```python
from build123d import *

# Parameters (mm, degrees)
EXTRUDE_THIN1_DEPTH = 10
FILLET1_R           = 0.5


with BuildPart() as part:
    # Sketch1 → Extrude-Thin1 (new body)
    with BuildSketch(Plane(origin=(0, 0, 0), x_dir=(1, 0, 0), z_dir=(0, 1, 0))):
        with BuildLine():
            ThreePointArc((31.228009552, -30.556896247), (17.805759331, -35.661082732), (3.450021006, -36.010793734))
            ThreePointArc((3.450021006, -36.010793734), (0.781528732, -34.960126351), (-1.143442514, -32.834276246))
            Line((-1.143442514, -32.834276246), (-11.514158233, -14.115081405))
            ThreePointArc((-11.514158233, -14.115081405), (-11.864920764, -12.594591782), (-11.35681344, -11.119210477))
            Line((-11.35681344, -11.119210477), (0, 5.1))
            Line((0, 5.1), (0, 0))
            Line((0, 0), (30, 0))
            Line((30, 0), (30, 5.1))
            Line((30, 5.1), (36.395958363, 2.511232605))
            ThreePointArc((36.395958363, 2.511232605), (37.463728778, 1.925417586), (38.366240646, 1.107624688))
            Line((38.366240646, 1.107624688), (42.902523658, -4.091619145))
            ThreePointArc((42.902523658, -4.091619145), (43.590417547, -5.096663868), (44.026071732, -6.233993339))
            Line((44.026071732, -6.233993339), (45.723869414, -12.921854211))
            ThreePointArc((45.723869414, -12.921854211), (45.883457457, -14.129266548), (45.7582513, -15.340726954))
            Line((45.7582513, -15.340726954), (44.251223786, -22.074141249))
            ThreePointArc((44.251223786, -22.074141249), (43.848071102, -23.223393532), (43.189020782, -24.247583736))
            Line((43.189020782, -24.247583736), (38.802344779, -29.573658617))
            ThreePointArc((38.802344779, -29.573658617), (37.883123065, -30.501625481), (36.810104599, -31.246422387))
            Line((36.810104599, -31.246422387), (28.716751538, -35.827648886))
            ThreePointArc((28.716751538, -35.827648886), (23.339920043, -38.206219709), (17.601311476, -39.485394366))
            ThreePointArc((17.601311476, -39.485394366), (9.20703571, -39.890619172), (0.842295428, -39.078712278))
            Line((0.842295428, -39.078712278), (1.179197641, -37.107292257))
            ThreePointArc((1.179197641, -37.107292257), (9.255554358, -37.891207773), (17.360428291, -37.499953535))
            ThreePointArc((17.360428291, -37.499953535), (22.714760553, -36.306436666), (27.731541539, -34.087142851))
            Line((27.731541539, -34.087142851), (35.824894599, -29.505916352))
            ThreePointArc((35.824894599, -29.505916352), (36.597062561, -28.969943927), (37.258554958, -28.302158326))
            Line((37.258554958, -28.302158326), (41.645230962, -22.976083445))
            ThreePointArc((41.645230962, -22.976083445), (42.051182062, -22.345219415), (42.299509498, -21.63732168))
            Line((42.299509498, -21.63732168), (43.806537012, -14.903907385))
            ThreePointArc((43.806537012, -14.903907385), (43.883659464, -14.157691701), (43.785359016, -13.413969481))
            Line((43.785359016, -13.413969481), (42.087561335, -6.72610861))
            ThreePointArc((42.087561335, -6.72610861), (41.819214153, -6.025554893), (41.39549646, -5.406483786))
            Line((41.39549646, -5.406483786), (36.859213448, -0.207239953))
            ThreePointArc((36.859213448, -0.207239953), (36.303298861, 0.29649082), (35.645591002, 0.657331631))
            Line((35.645591002, 0.657331631), (32, 2.13288644))
            Line((32, 2.13288644), (32, -2))
            Line((32, -2), (-2, -2))
            Line((-2, -2), (-2, -1.243189605))
            Line((-2, -1.243189605), (-9.718509351, -12.26636335))
            ThreePointArc((-9.718509351, -12.26636335), (-9.867673478, -12.69948831), (-9.764700771, -13.145855637))
            Line((-9.764700771, -13.145855637), (0.606014947, -31.865050477))
            ThreePointArc((0.606014947, -31.865050477), (1.919083649, -33.31514343), (3.73932574, -34.031828659))
            ThreePointArc((3.73932574, -34.031828659), (17.420438321, -33.698551784), (30.211930629, -28.834228658))
            Line((30.211930629, -28.834228658), (31.228009552, -30.556896247))
        make_face()
    extrude(amount=EXTRUDE_THIN1_DEPTH)

    # Fillet1
    fillet1_edges = [part.edges().sort_by_distance(p)[0] for p in [
        (0, 5, -5.1),
        (30, 5, -5.1),
    ]]
    fillet(fillet1_edges, radius=FILLET1_R)


solid = part.part
```
Read the model definition and answer for the solid it produces. Units are mm, in the model's axes. A direction names the side the tool comes from. Coordinates: 2 decimals unless noted, no trailing zeros. Loops run counter-clockwise (first coordinate to the right, second up) from the corner with the lowest first, then second, coordinate; pieces in that order, holes last. Notation, with made-up numbers: (41, 5.5) -> (93, 5.5) arc R14 ccw to (93, 15.5) -> close; hole circle Ø4 at (84, 20). An arc over 180 degrees is marked (long way). Return JSON: item names as keys, results as strings.
Item 1: Find section A-A (x = 6.5). Determine the outline of the cut face in (y, z), plus the area to 3 significant figures.
Answers:
{"outline": "(0, 0) -> (10, 0) -> (10, 2) -> (0, 2) -> close; (0, 34.34) -> (10, 34.34) -> (10, 36.34) -> (0, 36.34) -> close; (0, 37.76) -> (10, 37.76) -> (10, 39.76) -> (0, 39.76) -> close", "area": "60.1 mm2"}
Item 2: Find section B-B (z = 17). Determine the outline of the cut face in (x, y), plus the area to 3 significant figures.
Answers:
{"outline": "(-9.92, 0) -> (-7.63, 0) -> (-7.63, 10) -> (-9.92, 10) -> close; (43.34, 0) -> (45.39, 0) -> (45.39, 10) -> (43.34, 10) -> close", "area": "43.4 mm2"}
Item 3: Find section C-C (x = -4). Determine the outline of the cut face in (y, z).
Answers:
{"outline": "(0, 0.61) -> (10, 0.61) -> (10, 4.1) -> (0, 4.1) -> close; (0, 23.55) -> (10, 23.55) -> (10, 27.68) -> (0, 27.68) -> close"}
Item 4: For a pull along X with two mould halves and no side action, classify faces 1 (the flat face through (24, 10, 32)), 2 (the flat face through (43.04, 4.93, 18.32)), 3 (the cylindrical face through (37.45, 4.93, -1.935)) as +X half, -X half, draft (parallel to the pull), parting line (faces both ways), or undercut.
Answers:
{"face 1": "draft", "face 2": "undercut", "face 3": "+X half"}
Item 5: Find the intervals of material crossed by probe 1 along Z at (x, y) = (9.5, 4.75); probe 2 along Z at (x, y) = (20, 6.75); probe 3 along Z at (x, y) = (-5, 3.5), in increasing order.
Answers:
{"probe 1": "z = 0 to 2, 34.46 to 36.46, 37.9 to 39.9", "probe 2": "z = 0 to 2, 33.1 to 35.17, 37.05 to 39.09", "probe 3": "z = 2.04 to 5.53, 21.75 to 25.87"}
Item 6: Flat-ended cylindrical pins translate along their axes: P1, Ø3.5, axis at y = 3.5, z = -0.5, coming from the +X side; P2, Ø8, axis at x = 15.5, z = 26, coming from the +Y side; P3, Ø3, axis at x = 18.5, y = 3.5, coming from the +Z side; P4, Ø1.8, axis at y = 5, z = -1, coming from the +X side. Find the tip coordinate at first contact, or state that the pin passes through.
Answers:
{"P1": "stops at x = 40.42", "P2": "passes through", "P3": "stops at z = 39.56", "P4": "stops at x = 39.25"}
Item 7: For faces 4 (the cylindrical face through (9.325, 4.93, 39.893)), 5 (the flat face through (39.4, 4.9, 25.7)), 6 (the flat face through (1.008, 4.93, 38.107)), 7 (the flat face through (-6.256, 4.93, 23.606)), 8 (the flat face through (0, 5, -2)), determine the directions among +Z, -Z, +X, -X, +Y, -Y from which every point of the face is accessible in a straight line to the end or side of a thin tool.
Answers:
{"face 4": "+Z, +Y, -Y", "face 5": "+Y, -Y", "face 6": "-X, +Y, -Y", "face 7": "+Z, -X, +Y, -Y", "face 8": "-Z, +Y, -Y"}
